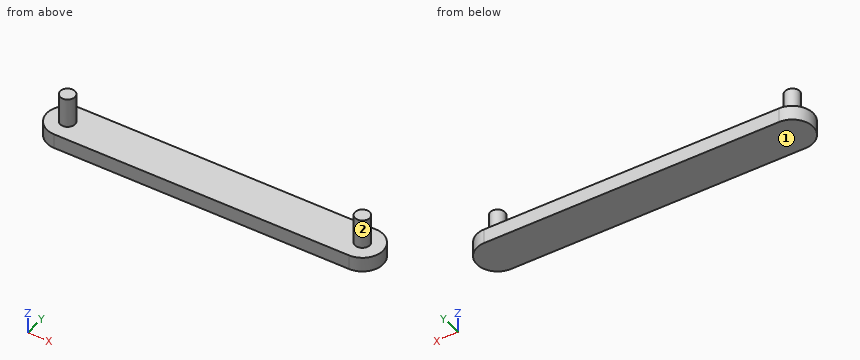
```python
from build123d import *

# Parameters (mm, degrees)
BOSS_EXTRUDE1_DEPTH = 5
SKETCH2_R           = 2.5
BOSS_EXTRUDE2_DEPTH = 10


with BuildPart() as part:
    # Sketch1 → Boss-Extrude1 (new body)
    with BuildSketch(Plane.XY):
        with BuildLine():
            Line((-50.000002608, -7.000000122), (50.000000869, -7.000000122))
            ThreePointArc((50.000000869, -7.000000122), (57.000000869, -1.22e-07), (50.000000869, 6.999999878))
            Line((50.000000869, 6.999999878), (-49.999999131, 6.999999878))
            ThreePointArc((-49.999999131, 6.999999878), (-57.000000869, 1.617e-06), (-50.000002608, -7.000000122))
        make_face()
    extrude(amount=BOSS_EXTRUDE1_DEPTH)

    # Sketch2 → Boss-Extrude2 (add)
    with BuildSketch(Plane.XY.offset(5)):
        with Locations(Location((-50.000000869, -1.22e-07, 0), (0, 0, 180))):
            Circle(SKETCH2_R)
        with Locations(Location((50.000000869, -1.22e-07, 0), (0, 0, 180))):
            Circle(SKETCH2_R)
    extrude(amount=BOSS_EXTRUDE2_DEPTH)


solid = part.part
```
The model under review builds one solid part; all positions refer to its coordinate system, in mm. Face numbers are marked on the shaded views. Coordinates: 2 decimals unless noted, no trailing zeros. Write each loop counter-clockwise with the first axis right and the second up, starting at its lowest first coordinate (ties: lowest second). Pieces come first, ordered by that corner, then holes. Notation, with made-up numbers: (43.5, 23.25) -> (83.5, 23.25) arc R16 cw to (83.5, 35.25) -> close; hole circle Ø9 at (-31, 41.25). An arc over 180 degrees is marked (long way). One line per item, written item: value. Start each with the question number.
Q1. The part is to be moulded in two halves that separate along X. For the marked faces 1 and 2, say which applies: +X half, -X half, draft (parallel to the pull), parting line (faces both ways), or undercut.
Q2. Add section B-B, the plane z = 6.5. Give the boundary of the cut face in (x, y), then the cut area to 3 significant figures.
Q3. Add section A-A, the plane y = 0. Give the boundary of the cut face in (x, z), then the cut area to 3 significant figures.
Q4. Add section C-C, the plane x = -18.5. Give the boundary of the cut face in (y, z).
Q5. To check wall thickness, follow probe 1 along X at (y, z) = (-2.25, 11.25); probe 2 along Z at (x, y) = (-34, -2.25); probe 3 along X at (y, z) = (-4.25, 3.75). State the ranges of each line that lie inside material, in increasing order.
Q6. Clearance check with flat-ended pins moving along their axes: P1, Ø8, axis at y = 4.5, z = 12.5, coming from the +X side; P2, Ø4, axis at x = 17.5, y = 1, coming from the +Z side; P3, Ø6, axis at x = -45, z = 9, coming from the +Y side. State where each tip first meets the part, or that it passes through.
Q7. Add section D-D, the plane z = 2.25. Give the boundary of the cut face in (x, y).
Response:
1. face 1: draft
1. face 2: undercut
2. outline: circle Ø5 at (-50, 0); circle Ø5 at (50, 0)
2. area: 39.3 mm²
3. outline: (-57, 0) -> (57, 0) -> (57, 5) -> (52.5, 5) -> (52.5, 15) -> (47.5, 15) -> (47.5, 5) -> (-47.5, 5) -> (-47.5, 15) -> (-52.5, 15) -> (-52.5, 5) -> (-57, 5) -> close
3. area: 670 mm²
4. outline: (-7, 0) -> (7, 0) -> (7, 5) -> (-7, 5) -> close
5. probe 1: -51.09 to -48.91, 48.91 to 51.09
5. probe 2: 0 to 5
5. probe 3: -55.56 to 55.56
6. P1: x = 52.45
6. P2: z = 5
6. P3: y = 1.5
7. outline: (-50, -7) -> (50, -7) arc R7 ccw to (50, 7) -> (-50, 7) arc R7 ccw to start
